```python
from build123d import *

# Parameters (mm, degrees)
SKETCH1_W           = 139.7
SKETCH1_H           = 149.225
BOSS_EXTRUDE1_DEPTH = 85.725
SKETCH2_W           = 47.625
SKETCH2_H           = 22.225
BOSS_EXTRUDE2_DEPTH = 6.35
SKETCH3_R           = 15.875
BOSS_EXTRUDE3_DEPTH = 6.35
SKETCH4_R           = 1.5875
CUT_EXTRUDE1_DEPTH  = 6.35


with BuildPart() as part:
    # Sketch1 → Boss-Extrude1 (new body)
    with BuildSketch(Plane(origin=(0, 0, 0), x_dir=(1, 0, 0), z_dir=(0, 1, 0))):
        with Locations((69.85, 74.6125)):
            Rectangle(SKETCH1_W, SKETCH1_H)
    extrude(amount=BOSS_EXTRUDE1_DEPTH)

    # Sketch2 → Boss-Extrude2 (add)
    with BuildSketch(Plane.ZY):
        with Locations((-30.1625, 42.8625)):
            Rectangle(SKETCH2_W, SKETCH2_H)
    extrude(amount=BOSS_EXTRUDE2_DEPTH)

    # Sketch3 → Boss-Extrude3 (add)
    with BuildSketch(Plane(origin=(139.7, 0, 0), x_dir=(0, 0, -1), z_dir=(1, 0, 0))):
        with Locations(Location((15.875, 42.8625, 0), (0, 0, 180))):
            Circle(SKETCH3_R)
    extrude(amount=BOSS_EXTRUDE3_DEPTH)

    # Sketch4 → Cut-Extrude1 (cut)
    with BuildSketch(Plane.ZY):
        with Locations((-6.35, 79.375)):
            Circle(SKETCH4_R)
        with Locations((-142.875, 79.375)):
            Circle(SKETCH4_R)
        with Locations((-142.875, 15.875)):
            Circle(SKETCH4_R)
        with Locations((-30.1625, 6.35)):
            Circle(SKETCH4_R)
    extrude(amount=-CUT_EXTRUDE1_DEPTH, mode=Mode.SUBTRACT)


solid = part.part
```
CAD build for the part. Positions are in the model's coordinates, mm. A direction names the side the tool comes from. Coordinates: 2 decimals unless noted, no trailing zeros. Write each loop counter-clockwise with the first axis right and the second up, starting at its lowest first coordinate (ties: lowest second). Pieces come first, ordered by that corner, then holes. Notation, with made-up numbers: (16.5, 83.25) -> (72.5, 83.25) arc R14 cw to (72.5, 103.25) -> close; hole circle Ø4 at (88.5, 19.5). An arc over 180 degrees is marked (long way). Return JSON: item names as keys, results as strings. Group by question number.
Q1. Cut at A-A, the plane z = -37. Give the cut face in (x, y) (3 decimals), then the cut area to 3 significant figures.
Q2. Drill centre lines: line 1 (Y direction, x = 3.75, z = -6.35) (1 decimal); line 2 (Z direction, x = 3, y = 6) (3 decimals); line 3 (X direction, y = 52, z = -41.5). Where is each one in solid material? Low to high.
Q3. Flat gauge pins, fed straight in: pin 1 (2.5 mm diameter, centred on y = 15.5, z = -143, fed in from -X); pin 2 (7 mm diameter, centred on x = -4.5, y = 47, fed in from +Z); pin 3 (3.5 mm diameter, centred on y = 79.375, z = -142.875, fed in from +X); pin 4 (12 mm diameter, centred on x = 88, y = 14, fed in from +Z). Where does each tip first touch, or does it go through?
Q4. Cut at B-B, the plane y = 64. Give the cut face in (x, z) (3 decimals).
Q5. Cut at C-C, the plane z = -132. Give the cut face in (x, y) (3 decimals).
Q6. Which spindle directions (+Z, -Z, +X, -X, +Y, -Y) get a long thin tool onto all of the face, cutting with end or side? Do faces 1 (the face through (-3, 43, -53.975)), 2 (the face through (-3, 43, -6.35)), 3 (the face through (142.831, 38.094, -0.733)). Say none if no direction does.
Returned:
{
 "1": {"outline": "(-6.35, 31.75) -> (0, 31.75) -> (0, 0) -> (139.7, 0) -> (139.7, 85.725) -> (0, 85.725) -> (0, 53.975) -> (-6.35, 53.975) -> close", "area": "12,100 mm2"},
 "2": {"line 1": "y = 0 to 77.8, 81 to 85.7", "line 2": "z = -149.225 to -31.711, -28.614 to 0", "line 3": "x = -6.35 to 139.7"},
 "3": {"pin 1": "stops at x = 0", "pin 2": "stops at z = -6.35", "pin 3": "stops at x = 139.7", "pin 4": "stops at z = 0"},
 "4": {"outline": "(0, -149.225) -> (139.7, -149.225) -> (139.7, 0) -> (0, 0) -> close"},
 "5": {"outline": "(0, 0) -> (139.7, 0) -> (139.7, 85.725) -> (0, 85.725) -> close"},
 "6": {"face 1": "-Z, -X, +Y, -Y", "face 2": "+Z, -X, +Y, -Y", "face 3": "+X"}
}
